Build history of the part. All positions in model axes, mm. A direction names the side the tool comes from. Round coordinates to 2 decimals unless told otherwise and drop trailing zeros. Write each loop counter-clockwise with the first axis right and the second up, starting at its lowest first coordinate (ties: lowest second). Pieces come first, ordered by that corner, then holes.
Autodesk Inventor part; units mm, degrees
ref_plane "YZ Plane" through (0, 0, 0) normal (1, 0, 0) x (0, 1, 0)
ref_plane "XZ Plane" through (0, 0, 0) normal (0, 1, 0) x (-1, 0, 0)
ref_plane "XY Plane" through (0, 0, 0) normal (0, 0, 1) x (1, 0, 0)
sketch "スケッチ1" plane through (0, 0, 0) normal (0, 1, 0) x (-1, 0, 0)
  line L0 (0, 0) -> (4, 0)
  line L1 (4, 0) -> (4, 10)
  line L2 (4, 10) -> (0, 10)
  line L3 (0, 10) -> (0, 0)
  dimension "d0" = 4
  dimension "d1" = 10
extrude "押し出し1" add sketch "スケッチ1" along normal blind 3.7
sketch "スケッチ2" plane through (-4, 0, 10) normal (0, 0, 1) x (1, 0, 0)
  line L0 (0, 0) -> (0, 3.7)
  line L1 (0, 2.7) -> (2.7, 2.7)
  line L2 (2.7, 2.7) -> (2.7, 1)
  line L3 (2.7, 1) -> (0, 1)
  line L4 (0, 1) -> (0, 2.7)
  point P0 (4, 0)
  point P1 (0, 1.85)
  dimension "d4" = 2.7
  dimension "d5" = 1.7
extrude "押し出し2" cut sketch "スケッチ2" against normal through all
sketch "スケッチ3" plane through (0, 0, 10) normal (1, 0, 0) x (0, 0, -1)
  line L0 (0, 0) -> (10, 0)
  line L1 (0, 3.7) -> (10, 3.7)
  circle A0 centre (8.15, 1.85) radius 1.85
  line L2 (10, 0) -> (10, 3.7)
  circle A1 centre (8.15, 1.85) radius 1.5
  dimension "d8" = 3
extrude "押し出し3" add sketch "スケッチ3" along normal blind 3 contours A1
sketch "スケッチ4" plane through (0, 3.7, 0) normal (0, 1, 0) x (1, 0, 0)
  line L0 (0, -10) -> (0, 0)
  line L1 (0, 0) -> (-4, 0)
  line L2 (-4, 0) -> (-4, -10)
  circle A0 centre (-2, -2) radius 0.8
  circle A1 centre (-2, -8) radius 2 construction
  line L3 (-4, -10) -> (0, -10)
  circle A2 centre (-2, -8) radius 0.8
  dimension "d15" = 1.6
  dimension "d18" = 1.6
extrude "押し出し4" cut sketch "スケッチ4" against normal through all contours A0 | A2
properties part number "chest_cover_axis_right"
1) Slice it at C-C (y = 0.65). Write the cut outline in (x, z).
Results:
outline: (-4, 0) - (0, 0) - (0, 0.95) - (3, 0.95) - (3, 2.75) - (0, 2.75) - (0, 10) - (-4, 10) - close; hole circle Ø1.6 at (-2, 2); hole circle Ø1.6 at (-2, 8)
2) Mould opens along X. For faces 1 (the flat face through (3, 2, 2)), 2 (the flat face through (-2, 0, 5)), 3 (the cylindrical face through (-1.237, 1.876, 1.76)) say: released by +X, released by -X, zero draft, split by the parting line, or undercut.
Results:
face 1: released by +X
face 2: zero draft
face 3: undercut
3) Slice it at B-B (z = 8). Write the cut outline in (x, y).
Results:
outline: (-4, 0) - (-2.8, 0) - (-2.8, 1) - (-4, 1) - close; (-4, 2.7) - (-2.8, 2.7) - (-2.8, 3.7) - (-4, 3.7) - close; (-1.2, 0) - (0, 0) - (0, 3.7) - (-1.2, 3.7) - close
4) Pin check, flat tips, straight feed: pin 1 Ø1.3 at (x, z) = (-2, 8) entering from -Y; pin 2 Ø1.5 at (x, y) = (2, 1.5) entering from +Z; pin 3 Ø4 at (x, z) = (1.5, 8.5) entering from +Y; pin 4 Ø1 at (x, y) = (1, 2) entering from -Z. Stop position of each tip, or through.
Results:
pin 1: passes through
pin 2: stops at z = 3.35
pin 3: stops at y = 3.7
pin 4: stops at z = 0.35
5) Wall check: L1, parallel to Z at x = -2, y = 3; L2, parallel to X at y = 0.5, z = 8; L3, parallel to Y at x = -1.5, z = 4. Give the ranges that are in metal, low to high.
Results:
L1: z = 0 to 1.2, 2.8 to 7.2, 8.8 to 10
L2: x = -4 to -2.8, -1.2 to 0
L3: y = 0 to 1, 2.7 to 3.7
6) Which spindle directions (+Z, -Z, +X, -X, +Y, -Y) get a long thin tool onto all of the face, cutting with end or side? Do faces 4 (the flat face through (-1.3, 2, 1)), 5 (the flat face through (-1, 2, 10)), 6 (the cylindrical face through (1.479, 3.314, 2.175)). Say none if no direction does.
Results:
face 4: +Z, -Z, -X
face 5: +Z, +X, -X, +Y, -Y
face 6: +X
7) Slice it at D-D (z = 5.5). Write the cut outline in (x, y).
Results:
outline: (-4, 0) - (0, 0) - (0, 3.7) - (-4, 3.7) - (-4, 2.7) - (-1.3, 2.7) - (-1.3, 1) - (-4, 1) - close
8) Slice it at A-A (x = -2). Write the cut outline in (y, z).
Results:
outline: (0, 0) - (1, 0) - (1, 1.2) - (0, 1.2) - close; (0, 2.8) - (1, 2.8) - (1, 7.2) - (0, 7.2) - close; (0, 8.8) - (1, 8.8) - (1, 10) - (0, 10) - close; (2.7, 0) - (3.7, 0) - (3.7, 1.2) - (2.7, 1.2) - close; (2.7, 2.8) - (3.7, 2.8) - (3.7, 7.2) - (2.7, 7.2) - close; (2.7, 8.8) - (3.7, 8.8) - (3.7, 10) - (2.7, 10) - close
